The model under review builds one solid part; all positions refer to its coordinate system, in mm. Face numbers are marked on the shaded views. A direction names the side the tool comes from. Give positions to 0.01 mm unless a question says otherwise; leave off trailing zeros. Write each loop counter-clockwise with the first axis right and the second up, starting at its lowest first coordinate (ties: lowest second). Pieces come first, ordered by that corner, then holes. Notation, with made-up numbers: (-30, 27.25) - (0, 27.25) arc R12 cw to (0, 33.25) - close; hole circle Ø6 at (8, 46). An arc over 180 degrees is marked (long way). Write item = value, one per line.
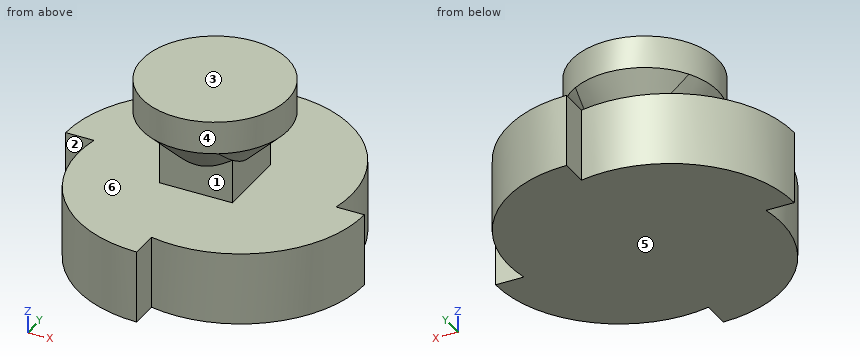
```python
from build123d import *

# Parameters (mm, degrees)
F0_W     = 41
F0_H     = 41
F0_W_2   = 10
F0_H_2   = 10
F1_DEPTH = 10
F2_DEPTH = 25
F3_R     = 10
F4_DEPTH = 8
F6_DEPTH = 25
F7_DEPTH = 1.5
F8_DEPTH = 3


# Not quite as in the source:
# - a fillet or chamfer that OpenCascade refuses, or shapes differently, is made with other operations: its cross-section is extruded or revolved along the edge and cut away or added


with BuildPart() as f1:
    # F0 (on Top) → F1 (new body)
    with BuildSketch(Plane.XY):
        Rectangle(F0_W, F0_H)
        Rectangle(F0_W_2, F0_H_2, mode=Mode.SUBTRACT)
        Rectangle(F0_W_2, F0_H_2)
    extrude(amount=F1_DEPTH)

    # F0 (on Top) → F2 (join)
    with BuildSketch(Plane.XY):
        Rectangle(F0_W_2, F0_H_2)
    extrude(amount=F2_DEPTH)

    # F3 (on face) → F4 (join)
    with BuildSketch(Plane.XY.offset(25)):
        Circle(F3_R)
    extrude(amount=-F4_DEPTH)

    # F5 (on face) → F6 (cut)
    with BuildSketch(Plane(origin=(0, 0, 0), x_dir=(1, 0, 0), z_dir=(0, 0, -1))):
        with BuildLine():
            Line((0, 20.5), (0, 16.625))
            ThreePointArc((0, 16.625), (14.2014511666, 13.1849661001), (20.5, 0))
            Line((20.5, 0), (20.5, 20.5))
            Line((20.5, 20.5), (0, 20.5))
        make_face()
        with BuildLine():
            Line((20.5, -20.5), (20.5, 0))
            Line((20.5, 0), (16.625, 0))
            ThreePointArc((16.625, 0), (13.15340166, -14.1758531755), (0, -20.5))
            Line((0, -20.5), (20.5, -20.5))
        make_face()
        with BuildLine():
            ThreePointArc((0, -16.625), (-14.1919455674, -13.1732449101), (-20.5, 0))
            Line((-20.5, 0), (-20.5, -20.5))
            Line((-20.5, -20.5), (0, -20.5))
            Line((0, -20.5), (0, -16.625))
        make_face()
        with BuildLine():
            ThreePointArc((-16.625, 0), (-13.1636820987, 14.1841903605), (0, 20.5))
            Line((0, 20.5), (-20.5, 20.5))
            Line((-20.5, 20.5), (-20.5, 0))
            Line((-20.5, 0), (-16.625, 0))
        make_face()
    extrude(amount=-F6_DEPTH, mode=Mode.SUBTRACT)

    # F7 (cut): a face of the model
    f7_faces = [f1.faces().sort_by_distance(p)[0] for p in [
        (0, 0, 25),
    ]]
    extrude(f7_faces, amount=-F7_DEPTH, mode=Mode.SUBTRACT)

    # F8 (add): a face of the model
    f8_faces = [f1.faces().sort_by_distance(p)[0] for p in [
        (-9.7171572875, 0, 17),
    ]]
    extrude(f8_faces, amount=F8_DEPTH)

    # F9: chamfer of 5 on 1 edges, made by hand


with BuildPart() as f9_tool2:
    # F9_s3 → F9_t4 (revolve)
    with BuildSketch(Plane.XZ):
        Polygon((5, 14), (10, 19), (10, 14), align=None)
    revolve(axis=Axis((0, 0, 14), (0, 0, 1)))

    split(bisect_by=Plane.YZ.offset(5), keep=Keep.TOP)


with BuildPart() as f1_1:
    add(f1.part)

    # F9_t1: cut F9_tool2
    add(f9_tool2.part, mode=Mode.SUBTRACT)


with BuildPart() as f9_tool7:
    # F9_s8 → F9_t9 (revolve)
    with BuildSketch(Plane.XZ):
        Polygon((5, 14), (10, 19), (10, 14), align=None)
    revolve(axis=Axis((0, 0, 14), (0, 0, 1)))

    split(bisect_by=Plane.XZ.offset(-5), keep=Keep.BOTTOM)


with BuildPart() as f1_2:
    add(f1_1.part)

    # F9_t6: cut F9_tool7
    add(f9_tool7.part, mode=Mode.SUBTRACT)


with BuildPart() as f9_tool12:
    # F9_s13 → F9_t14 (revolve)
    with BuildSketch(Plane.XZ):
        Polygon((5, 14), (10, 19), (10, 14), align=None)
    revolve(axis=Axis((0, 0, 14), (0, 0, 1)))

    split(bisect_by=Plane.YZ.offset(-5), keep=Keep.BOTTOM)


with BuildPart() as f1_3:
    add(f1_2.part)

    # F9_t11: cut F9_tool12
    add(f9_tool12.part, mode=Mode.SUBTRACT)


with BuildPart() as f9_tool17:
    # F9_s18 → F9_t19 (revolve)
    with BuildSketch(Plane.XZ):
        Polygon((5, 14), (10, 19), (10, 14), align=None)
    revolve(axis=Axis((0, 0, 14), (0, 0, 1)))

    split(bisect_by=Plane.XZ.offset(5), keep=Keep.TOP)


with BuildPart() as f1_4:
    add(f1_3.part)

    # F9_t16: cut F9_tool17
    add(f9_tool17.part, mode=Mode.SUBTRACT)


solid = f1_4.part
```
1. Take a section at A-A on z = 5.25. Give the boundary of the cut face in (x, y) (3 decimals).
Findings below:
outline = (-20.5, 0) - (-16.625, 0) arc R17.065 ccw to (0, -20.5) - (0, -16.625) arc R17.018 ccw to (20.5, 0) - (16.625, 0) arc R17.088 ccw to (0, 20.5) - (0, 16.625) arc R17.044 ccw to start
2. Draft analysis for pull direction Z (two halves, no side actions). For the marked faces 1, 2 and 3, state which applies: +Z half, -Z half, draft (parallel to the pull), parting line (faces both ways), or undercut.
Findings below:
face_1 = undercut
face_2 = draft
face_3 = +Z half
3. Take a section at C-C on x = -14.5. Give the boundary of the cut face in (y, z), and give its area (3 significant figures).
Findings below:
outline = (-12.29, 0) - (12.92, 0) - (12.92, 10) - (-12.29, 10) - close
area = 252 mm²
4. For line 1 (Z direction, x = 2, y = 14); line 2 (X direction, y = -4, z = 12.5); line 3 (Z direction, x = -7, y = 4.5), list the stretches that pass through material, from the lowest coordinate up. Write a range as from..to.
Findings below:
line_1 = 0..10
line_2 = -5..5
line_3 = 0..10, 17.32..23.5
5. Insertion check: P1, Ø3, axis at x = -6, y = -15.5, coming from the +Z side; P2, Ø6.5, axis at x = 0.5, z = 14.5, coming from the +Y side; P3, Ø8, axis at y = 6, z = 7.5, coming from the +X side. Each pin has a flat end and moves straight along its axis. Give the tip position at first contact, or say it passes through.
Findings below:
P1 = 10
P2 = 8.74
P3 = 16.97
6. Take a section at B-B on y = -11.5. Give the boundary of the cut face in (x, z).
Findings below:
outline = (-14.95, 0) - (16, 0) - (16, 10) - (-14.95, 10) - close
7. Machinability: for the marked faces 4, 5 and 6, which of the approach directions +Z, -Z, +X, -X, +Y, -Y give a long, thin tool a straight path to every point of the face, cutting with its end or side? Answer none if there is none.
Findings below:
face_4 = +Z
face_5 = -Z, +X, -X, +Y, -Y
face_6 = none
